Read the model definition and answer for the solid it produces. Units are mm, in the model's axes. Face numbers are marked on the shaded views. A direction names the side the tool comes from. Coordinates: 2 decimals unless noted, no trailing zeros. Write each loop counter-clockwise with the first axis right and the second up, starting at its lowest first coordinate (ties: lowest second). Pieces come first, ordered by that corner, then holes. Notation, with made-up numbers: (-36.5, 9) -> (-15.5, 9) arc R14 cw to (-15.5, 33) -> close; hole circle Ø4 at (6.5, -17.5). An arc over 180 degrees is marked (long way). One line per item, written item: value. Start each with the question number.
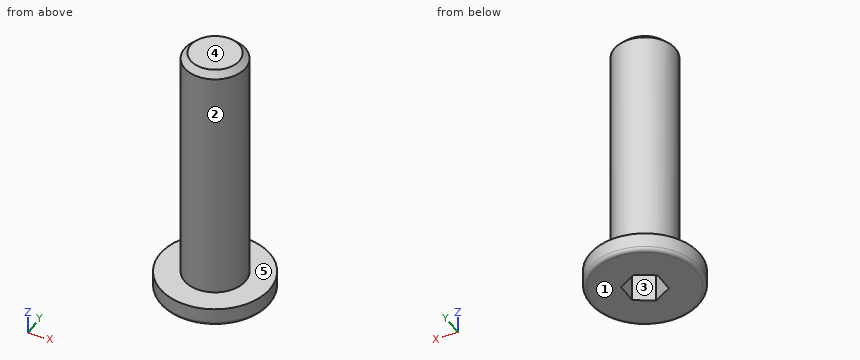
from build123d import *

# Parameters (mm, degrees)
F0_R      = 2.5
F1_DEPTH  = 20
F0_R_2    = 4.5
F1_FACE_R = 2.5
F2_DEPTH  = 1.5
F4_R      = 0.3
F5_DEPTH  = 3
F6_SIZE   = 0.5


with BuildPart() as f1:
    # F0 (on Top) → F1 (new body)
    with BuildSketch(Plane.XY):
        Circle(F0_R)
    extrude(amount=F1_DEPTH)

    # F0 (on Top) + F1_face (on face) → F2 (join)
    with BuildSketch(Plane.XY):
        Circle(F0_R_2)
        Circle(F0_R, mode=Mode.SUBTRACT)
    with BuildSketch(Plane(origin=(0, 0, 0), x_dir=(1, 0, 0), z_dir=(0, 0, -1))):
        Circle(F1_FACE_R)
    extrude(amount=-F2_DEPTH, dir=(0, 0, 1))

    # F4
    f4_edges = [f1.edges().sort_by_distance(p)[0] for p in [
        (-4.5, 0, -1.5),
    ]]
    fillet(f4_edges, radius=F4_R)

    # F3 (on face) → F5 (cut)
    with BuildSketch(Plane(origin=(0, 0, -1.5), x_dir=(1, 0, 0), z_dir=(0, 0, -1))):
        Polygon((-1.4980509352, -0.869392544), (0.0038905614, -1.732046438), (1.5019414966, -0.862653894), (1.4980509352, 0.869392544), (-0.0038905614, 1.732046438), (-1.5019414966, 0.862653894), align=None)
    extrude(amount=-F5_DEPTH, mode=Mode.SUBTRACT)

    # F6
    f6_edges = [f1.edges().sort_by_distance(p)[0] for p in [
        (-2.5, 0, 20),
    ]]
    chamfer(f6_edges, length=F6_SIZE)


solid = f1.part
1. Find the intervals of material crossed by probe 1 along X at (y, z) = (2, 13.5); probe 2 along Z at (x, y) = (-2.5, -3); probe 3 along X at (y, z) = (1.5, 3.25), in increasing order. Write a range as from..to.
2. A cutting plane is placed at B-B on z = 8.25. Give the vertices of the cut face in (x, y), then the cut area to 3 significant figures.
3. Given pin 1 (3 mm diameter, centred on x = 2.5, z = 16.5, fed in from +Y); pin 2 (3 mm diameter, centred on x = 3.5, z = 11.5, fed in from -Y); pin 3 (5 mm diameter, centred on y = 1, z = 14.5, fed in from +X), each flat-ended and moving along its own axis, determine where each tip first touches the part or whether it passes through.
4. A tool of negligible diameter and unlimited length cuts with its end or side. For the marked faces 4 and 5, from which of +Z, -Z, +X, -X, +Y, -Y can it reach the whole face along a straight path? Write none if from no direction.
5. A cutting plane is placed at A-A on y = 0. Give the vertices of the cut face in (x, z), then the cut area to 3 significant figures.
6. For a pull along Y with two mould halves and no side action, classify the marked faces 1, 2 and 3 as +Y half, -Y half, draft (parallel to the pull), parting line (faces both ways), or undercut.
Derived:
1. probe 1: x = -1.5..1.5
1. probe 2: z = -1.5..0
1. probe 3: x = -2..2
2. outline: circle Ø5 at (0, 0)
2. area: 19.6 mm2
3. pin 1: stops at y = 2.29
3. pin 2: stops at y = -1.5
3. pin 3: stops at x = 2.5
4. face 4: +Z, +X, -X, +Y, -Y
4. face 5: +Z
5. outline: (-4.5, -1.2) arc R0.3 ccw to (-4.2, -1.5) -> (-1.5, -1.5) -> (-1.5, 1.5) -> (1.5, 1.5) -> (1.5, -1.5) -> (4.2, -1.5) arc R0.3 ccw to (4.5, -1.2) -> (4.5, 0) -> (2.5, 0) -> (2.5, 19.5) -> (2, 20) -> (-2, 20) -> (-2.5, 19.5) -> (-2.5, 0) -> (-4.5, 0) -> close
5. area: 104 mm2
6. face 1: draft
6. face 2: parting line
6. face 3: undercut
